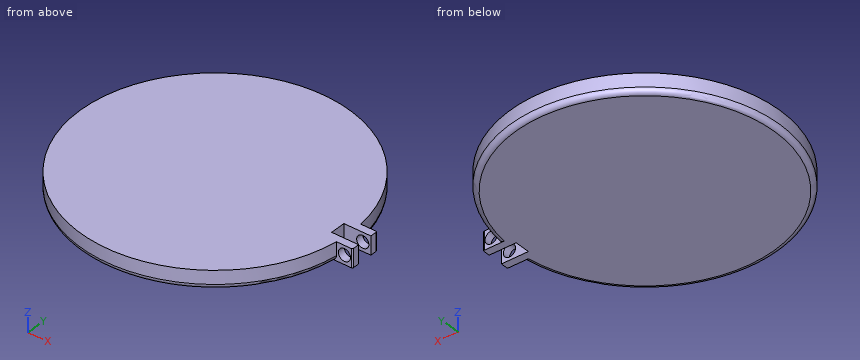
from build123d import *

# Parameters (mm, degrees)
SKETCH1_R               = 22
BOSS_EXTRUDE1_DEPTH     = 3
SKETCH2_W               = 5
SKETCH2_H               = 5
BOSS_EXTRUDE2_DEPTH     = 3
CUT_EXTRUDE1_DEPTH      = 35.777866525
CUT_EXTRUDE1_DEPTH_BACK = 35.777866525
SKETCH3_R               = 1
SKETCH4_W               = 3
SKETCH4_H               = 2.5
CUT_EXTRUDE2_DEPTH      = 2.6
FILLET1_R               = 0.2
FILLET2_R               = 0.8
SKETCH5_W               = 3
SKETCH5_H               = 2.5
CUT_EXTRUDE3_DEPTH      = 1.82


with BuildPart() as part:
    # Sketch1 → Boss-Extrude1 (new body)
    with BuildSketch(Plane.XY):
        Circle(SKETCH1_R)
    extrude(amount=BOSS_EXTRUDE1_DEPTH)

    # Sketch2 → Boss-Extrude2 (add)
    with BuildSketch(Plane.XY.offset(3)):
        with Locations((22, 0)):
            Rectangle(SKETCH2_W, SKETCH2_H)
    extrude(amount=-BOSS_EXTRUDE2_DEPTH)

    # Sketch3 → Cut-Extrude1 (cut, two sides: drawn at the far end of the back side and taken through both)
    with BuildSketch(Plane(origin=(0, 2.5, 0), x_dir=(1, 0, 0), z_dir=(0, 1, 0)).offset(-CUT_EXTRUDE1_DEPTH_BACK)):
        with Locations(Location((23.178746497, -1.5, 0), (0, 0, 270))):
            Circle(SKETCH3_R)
    extrude(amount=CUT_EXTRUDE1_DEPTH + CUT_EXTRUDE1_DEPTH_BACK, mode=Mode.SUBTRACT)

    # Sketch4 → Cut-Extrude2 (cut)
    with BuildSketch(Plane(origin=(24.5, 0, 0), x_dir=(0, 0, -1), z_dir=(1, 0, 0))):
        with Locations((-1.5, 0)):
            Rectangle(SKETCH4_W, SKETCH4_H)
    extrude(amount=-CUT_EXTRUDE2_DEPTH, mode=Mode.SUBTRACT)

    # Fillet1
    fillet1_edges = [part.edges().sort_by_distance(p)[0] for p in [
        (24.5, -2.5, 1.5),
        (24.5, 2.5, 1.5),
    ]]
    fillet(fillet1_edges, radius=FILLET1_R)

    # Fillet2
    fillet2_edges = [part.edges().sort_by_distance(p)[0] for p in [
        (-22, 0, 0),
    ]]
    fillet(fillet2_edges, radius=FILLET2_R)

    # Sketch5 → Cut-Extrude3 (cut)
    with BuildSketch(Plane(origin=(21.9, 0, 0), x_dir=(0, 0, -1), z_dir=(1, 0, 0))):
        with Locations((-1.5, 0)):
            Rectangle(SKETCH5_W, SKETCH5_H)
    extrude(amount=-CUT_EXTRUDE3_DEPTH, mode=Mode.SUBTRACT)


solid = part.part
Part model, mm, in its own coordinate system. Coordinates: 2 decimals unless noted, no trailing zeros. Write each loop counter-clockwise with the first axis right and the second up, starting at its lowest first coordinate (ties: lowest second). Pieces come first, ordered by that corner, then holes. Notation, with made-up numbers: (-24, -26.5) - (21, -26.5) arc R20 cw to (21, 7.5) - close; hole circle Ø6 at (56.5, 79). An arc over 180 degrees is marked (long way). Put each result on its own line as item: value.
1. Probe line 1 along X through (y, z) = (-1.8, 1.5); line 2 along X through (y, z) = (-1.45, 1.5); line 3 along X through (y, z) = (8, 1.45). List the from-to ranges inside material, lowest first. Write a range as [from, to].
Final values:
line 1: x = [-21.93, 22.18], [24.18, 24.5]
line 2: x = [-21.95, 22.18], [24.18, 24.5]
line 3: x = [-20.49, 20.49]
2. Band-saw the part on B-B (y = 0). Write the cut outline in (x, z).
Final values:
outline: (-22, 0.8) arc R0.8 ccw to (-21.2, 0) - (20.08, 0) - (20.08, 3) - (-22, 3) - close
3. Flat gauge pins, fed straight in: pin 1 Ø1.8 at (x, z) = (23.18, 1.5) entering from -Y; pin 2 Ø1.5 at (y, z) = (17.5, 2) entering from +X. Where does each tip first touch, or does it go through?
Final values:
pin 1: passes through
pin 2: stops at x = 14.26
4. Band-saw the part on A-A (z = 1.5). Write the cut outline in (x, y), then the cut area to 3 significant figures.
Final values:
outline: (20.08, -1.25) - (20.08, 1.25) - (22.18, 1.25) - (22.18, 2.5) - (21.86, 2.5) arc R22 ccw (long way) to (21.86, -2.5) - (22.18, -2.5) - (22.18, -1.25) - close; (24.18, -2.5) - (24.3, -2.5) arc R0.2 ccw to (24.5, -2.3) - (24.5, -1.25) - (24.18, -1.25) - close; (24.18, 1.25) - (24.5, 1.25) - (24.5, 2.3) arc R0.2 ccw to (24.3, 2.5) - (24.18, 2.5) - close
area: 1,520 mm²
